Design review of the part built by this model. Coordinates are the model's own, in mm. A direction names the side the tool comes from. Coordinates: 2 decimals unless noted, no trailing zeros. Write each loop counter-clockwise with the first axis right and the second up, starting at its lowest first coordinate (ties: lowest second). Pieces come first, ordered by that corner, then holes. Notation, with made-up numbers: (-2.75, 35.5) -> (13.25, 35.5) arc R16 ccw to (13.25, 40.5) -> close; hole circle Ø10 at (58.25, 67.25). An arc over 180 degrees is marked (long way). Answer in a Markdown table with one row per item. Add a question column.
Item 1: Take a section at B-B, the plane z = 5.5. Write out the cut boundary in (x, y), and give its area (3 significant figures).
Item 2: Take a section at C-C, the plane y = 25. Write out the cut boundary in (x, z).
Item 3: Take a section at D-D, the plane x = 85. Write out the cut boundary in (y, z), and give its area (3 significant figures).
Item 4: To check wall thickness, follow line 1 (Y direction, x = 124, z = -6.75); line 2 (Y direction, x = 80.5, z = 5.5); line 3 (Z direction, x = 164, y = 46). State the ranges of each line that lie inside material, in increasing order.
Item 5: For faces 4 (the face through (100, 15, 6)), 5 (the face through (24.8, 6.6, -4.9)), list the 3-axis set-ups (+Z, -Z, +X, -X, +Y, -Y) from which the entire face can be reached by the end or side of a thin tool; tool diameter is ignored.
Item 6: Take a section at A-A, the plane x = 108. Write out the cut boundary in (y, z).
Item 7: Clearance check with flat-ended pins moving along their axes: P1, Ø9.5, axis at y = 45, z = 6, coming from the -X side; P2, Ø10.5, axis at x = 156, y = 9, coming from the +Z side. State where each tip first meets the part, or that it passes through.
Item 8: Draft analysis for pull direction X (two halves, no side actions). For faces 1 (the face through (104, 9, -5)), 2 (the face through (75, 54, 6)), 3 (the face through (99, 95, -2)), state which applies: released by +X, released by -X, zero draft, split by the parting line, or undercut.
from build123d import *

# Parameters (mm, degrees)
F0_R     = 4
F0_W     = 50
F0_H     = 80
F0_R_2   = 3
F1_DEPTH = 10
F2_DEPTH = 12


with BuildPart() as f1:
    # F0 (on Top) → F1 (new body)
    with BuildSketch(Plane.XY):
        with BuildLine():
            Line((0, 85), (0, 0))
            Line((0, 0), (200, 0))
            Line((200, 0), (200, 85))
            ThreePointArc((200, 85), (197.071068, 92.071068), (190, 95))
            Line((190, 95), (125, 95))
            Line((125, 95), (125, 15))
            Line((125, 15), (75, 15))
            Line((75, 15), (75, 95))
            Line((75, 95), (10, 95))
            ThreePointArc((10, 95), (2.928932, 92.071068), (0, 85))
        make_face()
        with Locations((12, 9)):
            Circle(F0_R, mode=Mode.SUBTRACT)
        with Locations((28, 9)):
            Circle(F0_R, mode=Mode.SUBTRACT)
        with Locations((44, 9)):
            Circle(F0_R, mode=Mode.SUBTRACT)
        with Locations((60, 9)):
            Circle(F0_R, mode=Mode.SUBTRACT)
        with Locations((76, 9)):
            Circle(F0_R, mode=Mode.SUBTRACT)
        with Locations((92, 9)):
            Circle(F0_R, mode=Mode.SUBTRACT)
        with Locations((108, 9)):
            Circle(F0_R, mode=Mode.SUBTRACT)
        with Locations((124, 9)):
            Circle(F0_R, mode=Mode.SUBTRACT)
        with Locations((140, 9)):
            Circle(F0_R, mode=Mode.SUBTRACT)
        with Locations((156, 9)):
            Circle(F0_R, mode=Mode.SUBTRACT)
        with Locations((172, 9)):
            Circle(F0_R, mode=Mode.SUBTRACT)
        with Locations((188, 9)):
            Circle(F0_R, mode=Mode.SUBTRACT)
        with Locations((100, 55)):
            Rectangle(F0_W, F0_H)
        with Locations((85, 25)):
            Circle(F0_R_2, mode=Mode.SUBTRACT)
        with Locations((115, 25)):
            Circle(F0_R_2, mode=Mode.SUBTRACT)
        with Locations((85, 85)):
            Circle(F0_R_2, mode=Mode.SUBTRACT)
        with Locations((115, 85)):
            Circle(F0_R_2, mode=Mode.SUBTRACT)
    extrude(amount=-F1_DEPTH)

    # F0 (on Top) → F2 (join)
    with BuildSketch(Plane.XY):
        with Locations((100, 55)):
            Rectangle(F0_W, F0_H)
        with Locations((85, 25)):
            Circle(F0_R_2, mode=Mode.SUBTRACT)
        with Locations((115, 25)):
            Circle(F0_R_2, mode=Mode.SUBTRACT)
        with Locations((85, 85)):
            Circle(F0_R_2, mode=Mode.SUBTRACT)
        with Locations((115, 85)):
            Circle(F0_R_2, mode=Mode.SUBTRACT)
    extrude(amount=F2_DEPTH)


solid = f1.part
Answers:
| question | item | result |
|---|---|---|
| 1 | outline | (75, 15) -> (125, 15) -> (125, 95) -> (75, 95) -> close; hole circle Ø6 at (85, 25); hole circle Ø6 at (85, 85); hole circle Ø6 at (115, 25); hole circle Ø6 at (115, 85) |
| 1 | area | 3,890 mm^2 |
| 2 | outline | (0, -10) -> (82, -10) -> (82, 12) -> (75, 12) -> (75, 0) -> (0, 0) -> close; (88, -10) -> (112, -10) -> (112, 12) -> (88, 12) -> close; (118, -10) -> (200, -10) -> (200, 0) -> (125, 0) -> (125, 12) -> (118, 12) -> close |
| 3 | outline | (0, -10) -> (22, -10) -> (22, 12) -> (15, 12) -> (15, 0) -> (0, 0) -> close; (28, -10) -> (82, -10) -> (82, 12) -> (28, 12) -> close; (88, -10) -> (95, -10) -> (95, 12) -> (88, 12) -> close |
| 3 | area | 1,650 mm^2 |
| 4 | line 1 | y = 0 to 5, 13 to 95 |
| 4 | line 2 | y = 15 to 95 |
| 4 | line 3 | z = -10 to 0 |
| 5 | face 4 | +Z, +X, -X, -Y |
| 5 | face 5 | +Z, -Z |
| 6 | outline | (0, -10) -> (5, -10) -> (5, 0) -> (0, 0) -> close; (13, -10) -> (95, -10) -> (95, 12) -> (15, 12) -> (15, 0) -> (13, 0) -> close |
| 7 | P1 | stops at x = 75 |
| 7 | P2 | stops at z = 0 |
| 8 | face 1 | undercut |
| 8 | face 2 | released by -X |
| 8 | face 3 | zero draft |
